```python
from build123d import *

# Parameters (mm, degrees)
SKETCH1_R           = 46.99
BOSS_EXTRUDE1_DEPTH = 3.175
SKETCH2_R           = 14.351
CUT_EXTRUDE1_DEPTH  = 3.175
CUT_EXTRUDE2_START  = -5.08
SKETCH5_R           = 46.99
CUT_EXTRUDE2_DEPTH  = 5.08
CIRPATTERN1_COUNT   = 4


with BuildPart() as part:
    # Sketch1 → Boss-Extrude1 (new body)
    with BuildSketch(Plane(origin=(0, 0, 0), x_dir=(1, 0, 0), z_dir=(0, 1, 0))):
        with Locations(Location((0, 0, 0), (0, 0, 270))):
            Circle(SKETCH1_R)
    extrude(amount=BOSS_EXTRUDE1_DEPTH)

    # Sketch2 → Cut-Extrude1 (cut)
    with BuildSketch(Plane(origin=(0, 3.175, 0), x_dir=(1, 0, 0), z_dir=(0, 1, 0))):
        with Locations(Location((0, 0, 0), (0, 0, 270))):
            Circle(SKETCH2_R)
    extrude(amount=-CUT_EXTRUDE1_DEPTH, mode=Mode.SUBTRACT)

    # Sketch5 → Cut-Extrude2 (cut)
    with BuildSketch(Plane(origin=(0, 3.175, 0), x_dir=(1, 0, 0), z_dir=(0, 1, 0)).offset(CUT_EXTRUDE2_START)):
        Circle(SKETCH5_R)
        with BuildLine():
            Line((31.590851128, 3.175), (44.45, 3.175))
            Line((44.45, 3.175), (44.45, -3.175))
            Line((44.45, -3.175), (31.590851128, -3.175))
            ThreePointArc((31.590851128, -3.175), (22.450640303, -22.450640303), (3.175, -31.590851128))
            Line((3.175, -31.590851128), (3.175, -44.45))
            Line((3.175, -44.45), (-3.175, -44.45))
            Line((-3.175, -44.45), (-3.175, -31.590851128))
            ThreePointArc((-3.175, -31.590851128), (-22.450640303, -22.450640303), (-31.590851128, -3.175))
            Line((-31.590851128, -3.175), (-44.45, -3.175))
            Line((-44.45, -3.175), (-44.45, 3.175))
            Line((-44.45, 3.175), (-31.590851128, 3.175))
            ThreePointArc((-31.590851128, 3.175), (-22.450640303, 22.450640303), (-3.175, 31.590851128))
            Line((-3.175, 31.590851128), (-3.175, 44.45))
            Line((-3.175, 44.45), (3.175, 44.45))
            Line((3.175, 44.45), (3.175, 31.590851128))
            ThreePointArc((3.175, 31.590851128), (22.450640303, 22.450640303), (31.590851128, 3.175))
        make_face(mode=Mode.SUBTRACT)
    extrude(amount=CUT_EXTRUDE2_DEPTH, mode=Mode.SUBTRACT)

    # Sketch6 → #4 Clearance Hole1 (revolve, cut)
    with BuildSketch(Plane(origin=(0, 3.175, -38.1), x_dir=(0, 0, 1), z_dir=(1, 0, 0))):
        Polygon((0, 0), (0, 11.140574487), (1.63195, 10.16), (1.63195, 0), align=None)
    f_4_clearance_hole1 = revolve(axis=Axis((0, 9.525, -38.1), (0, -1, 0)), mode=Mode.SUBTRACT)

    # CirPattern1: #4 Clearance Hole1 ×4 about axis
    cirpattern1_axis = Axis((0, 0, 0), (0, 1, 0))
    for i in range(1, CIRPATTERN1_COUNT):
        add(f_4_clearance_hole1.rotate(cirpattern1_axis, i * 360 / CIRPATTERN1_COUNT), mode=Mode.SUBTRACT)


solid = part.part
```
CAD build for the part. Positions are in the model's coordinates, mm. A direction names the side the tool comes from. Coordinates: 2 decimals unless noted, no trailing zeros. Order: outer loops, then holes, each group sorted by start corner. A loop starts at its lowest first (then second) coordinate and runs counter-clockwise, first axis right, second up.
(1) Mould opens along X. For faces 1 (the face through (38, 2, -3.175)), 2 (the face through (-5.497, 1.61, 13.257)), 3 (the face through (3.175, 2, 38)) say: released by +X, released by -X, zero draft, split by the parting line, or undercut.
Solution:
face 1: zero draft
face 2: undercut
face 3: released by +X
(2) Saw through at A-A, the plane z = 38.1. Write the cut outline in (x, y) (3 decimals).
Solution:
outline: (-3.175, 0) - (-1.632, 0) - (-1.632, 3.175) - (-3.175, 3.175) - close; (1.632, 0) - (3.175, 0) - (3.175, 3.175) - (1.632, 3.175) - close
(3) Which spindle directions (+Z, -Z, +X, -X, +Y, -Y) get a long thin tool onto all of the face, cutting with end or side? Do faces 4 (the face through (-38, 2, 3.175)), 5 (the face through (38, 2, 3.175)), 6 (the face through (-3.175, 2, -38)), 7 (the face through (-44.45, 2, 0)), 8 (the face through (44.45, 2, 0)). Say none if no direction does.
Solution:
face 4: +Z, -X, +Y, -Y
face 5: +Z, +X, +Y, -Y
face 6: -Z, -X, +Y, -Y
face 7: +Z, -Z, -X, +Y, -Y
face 8: +Z, -Z, +X, +Y, -Y
(4) Pin check, flat tips, straight feed: pin 1 Ø3 at (x, z) = (0, -38.1) entering from -Y; pin 2 Ø5 at (x, z) = (0, 38.1) entering from -Y; pin 3 Ø1 at (x, y) = (40, 2) entering from +Z (3 decimals); pin 4 Ø1 at (x, y) = (-37.5, 1.5) entering from -Z (3 decimals). Stop position of each tip, or through.
Solution:
pin 1: passes through
pin 2: stops at y = 0
pin 3: stops at z = 3.175
pin 4: stops at z = -3.175
(5) Drill centre lines: L1, parallel to Z at x = -38, y = 0.95 (3 decimals); L2, parallel to X at y = 2, z = -38.1 (3 decimals); L3, parallel to Z at x = 40.5, y = 1.3 (3 decimals). Where is each one in solid material? Low to high.
Solution:
L1: z = -3.175 to -1.629, 1.629 to 3.175
L2: x = -3.175 to -1.632, 1.632 to 3.175
L3: z = -3.175 to 3.175
(6) Saw through at D-D, the plane y = 1.7. Write the cut outline in (x, z) (3 decimals), and give its area (3 significant figures).
Solution:
outline: (-44.45, -3.175) - (-31.591, -3.175) arc R31.75 ccw to (-3.175, -31.591) - (-3.175, -44.45) - (3.175, -44.45) - (3.175, -31.591) arc R31.75 ccw to (31.591, -3.175) - (44.45, -3.175) - (44.45, 3.175) - (31.591, 3.175) arc R31.75 ccw to (3.175, 31.591) - (3.175, 44.45) - (-3.175, 44.45) - (-3.175, 31.591) arc R31.75 ccw to (-31.591, 3.175) - (-44.45, 3.175) - close; hole circle Ø3.264 at (-38.1, 0); hole circle Ø28.702 at (0, 0); hole circle Ø3.264 at (0, -38.1); hole circle Ø3.264 at (0, 38.1); hole circle Ø3.264 at (38.1, 0)
area: 2,810 mm2
(7) Saw through at B-B, the plane x = 0. Write the cut outline in (y, z) (3 decimals), and give its area (3 significant figures).
Solution:
outline: (0, -44.45) - (3.175, -44.45) - (3.175, -39.732) - (0, -39.732) - close; (0, -36.468) - (3.175, -36.468) - (3.175, -14.351) - (0, -14.351) - close; (0, 14.351) - (3.175, 14.351) - (3.175, 36.468) - (0, 36.468) - close; (0, 39.732) - (3.175, 39.732) - (3.175, 44.45) - (0, 44.45) - close
area: 170 mm2
(8) Saw through at C-C, the plane z = 0. Write the cut outline in (x, y) (3 decimals), and give its area (3 significant figures).
Solution:
outline: (-44.45, 0) - (-39.732, 0) - (-39.732, 3.175) - (-44.45, 3.175) - close; (-36.468, 0) - (-14.351, 0) - (-14.351, 3.175) - (-36.468, 3.175) - close; (14.351, 0) - (36.468, 0) - (36.468, 3.175) - (14.351, 3.175) - close; (39.732, 0) - (44.45, 0) - (44.45, 3.175) - (39.732, 3.175) - close
area: 170 mm2
